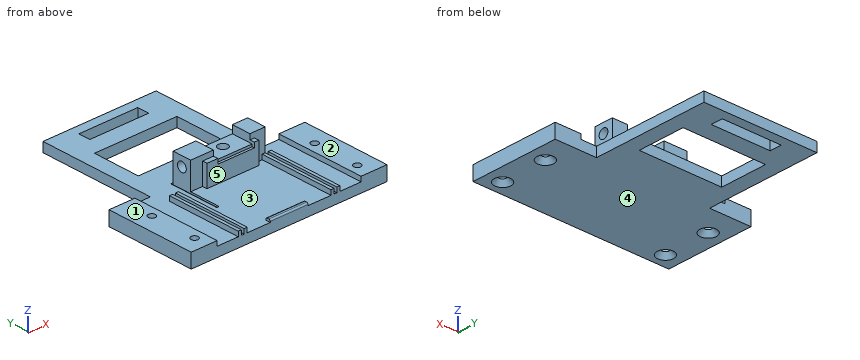
Solid Edge part; units mm, degrees
sketch "Sketch1" plane through (0, 0, 0) normal (0, 0, 1) x (1, 0, 0)
  line L0 (83.1, 37.5) -> (65.55, 37.5)
  line L1 (65.55, 37.5) -> (65.55, 86.5)
  line L2 (65.55, 86.5) -> (17.55, 86.5)
  line L3 (17.55, 86.5) -> (17.55, 37.5)
  line L4 (0, 37.5) -> (17.55, 37.5)
  line L5 (0, 0) -> (0, 37.5)
  line L6 (0, 0) -> (83.1, 0)
  line L7 (83.1, 0) -> (83.1, 37.5)
extrude "Protrusion1" add sketch "Sketch1" along normal blind 4
sketch "Sketch2" plane through (40.5, 43.25, 4) normal (0, 0, 1) x (1, 0, 0)
  line L0 (-29.5, -5.75) -> (-29.5, -43.25)
  line L1 (-29.5, -43.25) -> (-40.5, -43.25)
  line L2 (-40.5, -43.25) -> (-40.5, -5.75)
  line L3 (-40.5, -5.75) -> (-29.5, -5.75)
  line L4 (-20.53, -43.25) -> (-20.53, -11.85)
  line L5 (-20.53, -11.85) -> (-19.23, -11.85)
  line L6 (-19.23, -11.85) -> (-19.23, -43.25)
  line L7 (-19.23, -43.25) -> (-20.53, -43.25)
  line L8 (-16.73, -11.85) -> (-16.73, -43.25)
  line L9 (-16.73, -43.25) -> (-18.03, -43.25)
  line L10 (-18.03, -43.25) -> (-18.03, -11.85)
  line L11 (-18.03, -11.85) -> (-16.73, -11.85)
  line L12 (18.83, -11.85) -> (18.83, -43.25)
  line L13 (18.83, -43.25) -> (20.13, -43.25)
  line L14 (20.13, -43.25) -> (20.13, -11.85)
  line L15 (20.13, -11.85) -> (18.83, -11.85)
  line L16 (22.63, -43.25) -> (22.63, -11.85)
  line L17 (22.63, -11.85) -> (21.33, -11.85)
  line L18 (21.33, -11.85) -> (21.33, -43.25)
  line L19 (21.33, -43.25) -> (22.63, -43.25)
  line L20 (31.6, -5.75) -> (31.6, -43.25)
  line L21 (31.6, -43.25) -> (42.6, -43.25)
  line L22 (42.6, -43.25) -> (42.6, -5.75)
  line L23 (42.6, -5.75) -> (31.6, -5.75)
extrude "ExtrudedProtrusion_2" add sketch "Sketch2" along normal blind 2
sketch "Sketch3" plane through (41.55, 43.25, 4) normal (0, 0, 1) x (1, 0, 0)
  line L0 (-12.58, -11.85) -> (19.08, -11.85)
  line L1 (19.08, -11.85) -> (19.08, -3.85)
  line L2 (19.08, -3.85) -> (-12.58, -3.85)
  line L3 (-12.58, -11.85) -> (-12.58, -3.85)
extrude "ExtrudedProtrusion_3" add sketch "Sketch3" along normal blind 11.2
hole "Hole_1" at (60.63, 35.4, 11.2) direction (-1, 0, 0) diameter 4 depth 5.9
sketch "Sketch4" plane through (41.55, 43.25, 4) normal (0, 0, 1) x (1, 0, 0)
  line L0 (12.5, 34.25) -> (-12.5, 34.25)
  line L1 (-12.5, 34.25) -> (-12.5, 39.25)
  line L2 (-12.5, 39.25) -> (12.5, 39.25)
  line L3 (12.5, 39.25) -> (12.5, 34.25)
  line L4 (-17.5, 26.75) -> (17.5, 26.75)
  line L5 (17.5, 26.75) -> (17.5, 6.75)
  line L6 (17.5, 6.75) -> (-17.5, 6.75)
  line L7 (-17.5, 6.75) -> (-17.5, 26.75)
extrude "Cutout1" cut sketch "Sketch4" against normal through all
hole "Hole_3" at (7, 6, 0) direction (0, 0, 1) diameter 3 end through all countersink diameter 6.94 countersink angle 90
hole "Hole1" at (7, 25.5, 0) direction (0, 0, 1) diameter 3 end through all countersink diameter 6.94 countersink angle 90
hole "Hole2" at (76.1, 6, 0) direction (0, 0, 1) diameter 3 end through all countersink diameter 6.94 countersink angle 90
hole "Hole3" at (76.1, 25.5, 0) direction (0, 0, 1) diameter 3 end through all countersink diameter 6.94 countersink angle 90
sketch "Sketch5" plane through (41.55, 15.7, 4) normal (0, 0, 1) x (1, 0, 0)
  line L0 (-8.0007, -13.7) -> (7.9993, -13.7)
  line L1 (7.9993, -13.7) -> (7.9993, -15.7)
  line L2 (-8.0007, -15.7) -> (7.9993, -15.7)
  line L3 (-8.0007, -13.7) -> (-8.0007, -15.7)
extrude "ExtrudedProtrusion_4" add sketch "Sketch5" along normal blind 1
fillet "Round_1" radius 0.6 2 edges at (41.5493, 2, 5) (41.5493, 0, 5)
sketch "Sketch6" plane through (40.5, 43.25, 4) normal (0, 0, 1) x (1, 0, 0)
  line L0 (-11.53, -24.85) -> (-11.53, -11.85)
  line L1 (-11.53, -11.85) -> (-12.53, -11.85)
  line L2 (-12.53, -11.85) -> (-12.53, -24.85)
  line L3 (-12.53, -24.85) -> (-11.53, -24.85)
extrude "ExtrudedCutout_7" cut sketch "Sketch6" against normal blind 0.7
sketch "Sketch7" plane through (41.55, 35.4, 15.2) normal (0, 0, 1) x (1, 0, 0)
  line L0 (-13.58, 4) -> (-13.58, -4)
  line L1 (-13.58, -4) -> (-12.58, -4)
  line L2 (-12.58, -4) -> (-12.58, 4)
  line L3 (-12.58, 4) -> (-13.58, 4)
extrude "ExtrudedCutout_8" cut sketch "Sketch7" against normal blind 11.9
hole "Hole_7" at (28.97, 35.4, 11.2) direction (1, 0, 0) diameter 4 depth 6
sketch "Sketch8" plane through (44.8, 31.4, 9.6) normal (0, -1, 0) x (-1, 0, 0)
  line L0 (-11.23, -3.4) -> (-11.23, 5.6)
  line L1 (-11.23, 5.6) -> (10.77, 5.6)
  line L2 (10.77, 5.6) -> (10.77, -3.4)
  line L3 (10.77, -3.4) -> (-11.23, -3.4)
extrude "ExtrudedProtrusion_5" add sketch "Sketch8" along normal blind 2
sketch "Sketch9" plane through (44.8, 35.4, 15.2) normal (0, 0, 1) x (-1, 0, 0)
  line L0 (-9.33, -4.6) -> (-9.33, 7.4)
  line L1 (-9.33, 7.4) -> (6.17, 7.4)
  line L2 (6.17, 7.4) -> (6.17, -4.6)
  line L3 (6.17, -4.6) -> (-9.33, -4.6)
extrude "ExtrudedCutout_10" cut sketch "Sketch9" against normal blind 3.25
sketch "Sketch10" plane through (45.03, 29.4, 8.5) normal (0, -1, 0) x (-1, 0, 0)
  line L0 (6.4, -2.45) -> (-9.1, -2.45)
  line L1 (-9.1, -2.45) -> (-9.1, -3.45)
  line L2 (-9.1, -3.45) -> (6.4, -3.45)
  line L3 (6.4, -3.45) -> (6.4, -2.45)
extrude "ExtrudedCutout_11" cut sketch "Sketch10" against normal blind 1
hole "Hole_8" at (46.4, 35.4, 11.95) direction (0, 0, -1) diameter 4 depth 6
Model file for the job. Use its own axes, mm. Face numbers are marked on the shaded views. A direction names the side the tool comes from. Coordinates: 2 decimals unless noted, no trailing zeros. Loops run counter-clockwise (first coordinate to the right, second up) from the corner with the lowest first, then second, coordinate; pieces in that order, holes last. Notation, with made-up numbers: (3.25, -13.75) - (58.25, -13.75) arc R25 cw to (58.25, 17.25) - close; hole circle Ø1 at (19, 73). An arc over 180 degrees is marked (long way). Answer as a JSON object with one key per item and string values. Group by question number.
(1) Cut at B-B (y = 53). Give the cut face in (x, z), then the cut area to 3 significant figures.
(2) Tool access for the marked faces 1 and 2: list every direction of +Z, -Z, +X, -X, +Y, -Y with a clear straight run to the whole face (end or side of a thin tool).
(3) Cut at A-A (x = 46.4). Give the cut face in (y, z), then the cut area to 3 significant figures.
(4) Flat gauge pins, fed straight in: pin 1 (3.5 mm diameter, centred on x = 7, y = 25.5, fed in from -Z); pin 2 (9 mm diameter, centred on x = 75.5, y = 9.5, fed in from +Z); pin 3 (2 mm diameter, centred on y = 34.5, z = 13, fed in from +X). Where does each tip first touch, or does it go through?
(5) Two-plate mould, pull along X, no slides. Class the marked faces 3, 4 and 5: released by +X, released by -X, zero draft, split by the parting line, or undercut.
(6) Probe line 1 along Y through (x, z) = (7, 3.8); line 2 along Y through (x, z) = (45.5, 1.25); line 3 along X through (y, z) = (25.5, 3.9). List the from-to ranges inside material, lowest first.
(7) Cut at C-C (x = 7). Give the cut face in (y, z), then the cut area to 3 significant figures.
Geometry says:
{
 "1": {"outline": "(17.55, 0) - (24.05, 0) - (24.05, 4) - (17.55, 4) - close; (59.05, 0) - (65.55, 0) - (65.55, 4) - (59.05, 4) - close", "area": "52.0 mm^2"},
 "2": {"face 1": "+Z, -X, +Y, -Y", "face 2": "+Z, +X, +Y, -Y"},
 "3": {"outline": "(0, 0) - (50, 0) - (50, 4) - (39.4, 4) - (39.4, 11.95) - (37.4, 11.95) - (37.4, 5.95) - (33.4, 5.95) - (33.4, 11.95) - (30.4, 11.95) - (30.4, 10.95) - (29.4, 10.95) - (29.4, 4) - (2, 4) - (2, 4.4) arc R0.6 ccw to (1.4, 5) - (0.6, 5) arc R0.6 ccw to (0, 4.4) - close; (70, 0) - (77.5, 0) - (77.5, 4) - (70, 4) - close; (82.5, 0) - (86.5, 0) - (86.5, 4) - (82.5, 4) - close", "area": "302 mm^2"},
 "4": {"pin 1": "stops at z = 1.72", "pin 2": "stops at z = 6", "pin 3": "stops at x = 60.63"},
 "5": {"face 3": "undercut", "face 4": "zero draft", "face 5": "undercut"},
 "6": {"line 1": "y = 0 to 4.5, 7.5 to 24, 27 to 37.5", "line 2": "y = 0 to 50, 70 to 77.5, 82.5 to 86.5", "line 3": "x = 0 to 5.5, 8.5 to 27.97, 28.97 to 74.6, 77.6 to 83.1"},
 "7": {"outline": "(0, 0) - (2.53, 0) - (4.5, 1.97) - (4.5, 6) - (0, 6) - close; (7.5, 1.97) - (9.47, 0) - (22.03, 0) - (24, 1.97) - (24, 6) - (7.5, 6) - close; (27, 1.97) - (28.97, 0) - (37.5, 0) - (37.5, 6) - (27, 6) - close", "area": "181 mm^2"}
}
